Design review of the part built by this model. Coordinates are the model's own, in mm. Give positions to 0.01 mm unless a question says otherwise; leave off trailing zeros. Loops run counter-clockwise (first coordinate to the right, second up) from the corner with the lowest first, then second, coordinate; pieces in that order, holes last. Notation, with made-up numbers: M 68.25,43 L 87.25,43 A16 ccw 87.25,52 Z; hole C 51.25,-17.5 d9. An arc over 180 degrees is marked long. Use CSV: the item, a comma, the result in double quotes.
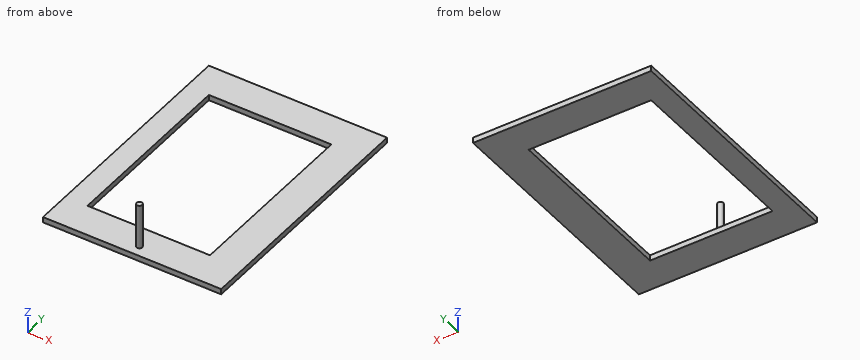
from build123d import *

# Parameters (mm, degrees)
F0_W     = 203.2
F0_H     = 25.4
F0_H_2   = 233.4768
F0_W_2   = 12.7
F0_H_3   = 182.6768
F0_H_4   = 12.7
F1_DEPTH = 6.35
F2_R     = 3.175
F3_DEPTH = 50.8


with BuildPart() as f1:
    # F0 (on Top) → F1 (new body)
    with BuildSketch(Plane.XY):
        with Locations((0, 129.4384)):
            Rectangle(F0_W, F0_H)
        with Locations((0, -129.4384)):
            Rectangle(F0_W, F0_H)
        Rectangle(F0_W, F0_H_2)
        Polygon((76.2, 91.3384), (76.2, -91.3384), (76.2, -104.0384), (63.5, -104.0384), (-63.5, -104.0384), (-76.2, -104.0384), (-76.2, -91.3384), (-76.2, 91.3384), (-76.2, 104.0384), (-63.5, 104.0384), (63.5, 104.0384), (76.2, 104.0384), align=None, mode=Mode.SUBTRACT)
        with Locations((69.85, 0)):
            Rectangle(F0_W_2, F0_H_3)
        with Locations((69.85, -97.6884)):
            Rectangle(F0_W_2, F0_H_4)
        with Locations((69.85, 97.6884)):
            Rectangle(F0_W_2, F0_H_4)
    extrude(amount=F1_DEPTH)

    # F2 (on face) → F3 (join)
    with BuildSketch(Plane.XY.offset(6.35)):
        with Locations((0, -129.4384)):
            Circle(F2_R)
    extrude(amount=F3_DEPTH)


solid = f1.part
(1) We need section A-A on x = -43. State the section outline as (y, z) points.
A:
outline,"M -142.14,0 L -104.04,0 L -104.04,6.35 L -142.14,6.35 Z; M 104.04,0 L 142.14,0 L 142.14,6.35 L 104.04,6.35 Z"
(2) We need section B-B on y = -18. State the section outline as (x, z) points, then the cut area to 3 significant figures.
A:
outline,"M -101.6,0 L -76.2,0 L -76.2,6.35 L -101.6,6.35 Z; M 63.5,0 L 101.6,0 L 101.6,6.35 L 63.5,6.35 Z"
area,"403 mm²"
(3) We need section D-D on y = -123. State the section outline as (x, z) points.
A:
outline,"M -101.6,0 L 101.6,0 L 101.6,6.35 L -101.6,6.35 Z"
(4) Clearance check with flat-ended pins moving along their axes: P1, Ø4, axis at x = 67, y = 71.5, coming from the +Z side; P2, Ø4, axis at x = 4, z = 26, coming from the -Y side. State where each tip first meets the part, or that it passes through.
A:
P1,"z = 6.35"
P2,"y = -131.9"
(5) Wall thickness on line 1 along Z through (x, y) = (71.5, 75.5); line 2 along Y through (x, z) = (2, 21): over which ranges is each line inside the solid? List them lowest first. Write a range as [from, to].
A:
line 1,"[0, 6.35]"
line 2,"[-131.9, -126.97]"
(6) We need section C-C on x = 0. State the section outline as (y, z) points.
A:
outline,"M -142.14,0 L -104.04,0 L -104.04,6.35 L -126.26,6.35 L -126.26,57.15 L -132.61,57.15 L -132.61,6.35 L -142.14,6.35 Z; M 104.04,0 L 142.14,0 L 142.14,6.35 L 104.04,6.35 Z"
